Print and shaded views of the part. All mm, measured from the part's lowest x, y and z. A direction names the side the tool comes from. Give positions to 0.01 mm unless a question says otherwise; leave off trailing zeros. Write each loop counter-clockwise with the first axis right and the second up, starting at its lowest first coordinate (ties: lowest second). Pieces come first, ordered by that corner, then holes. Notation, with made-up numbers: (-18, 83) -> (27, 83) arc R25 ccw to (27, 119) -> close; hole circle Ø10 at (25, 30). An arc over 180 degrees is marked (long way). Put each result on its own line as item: value.
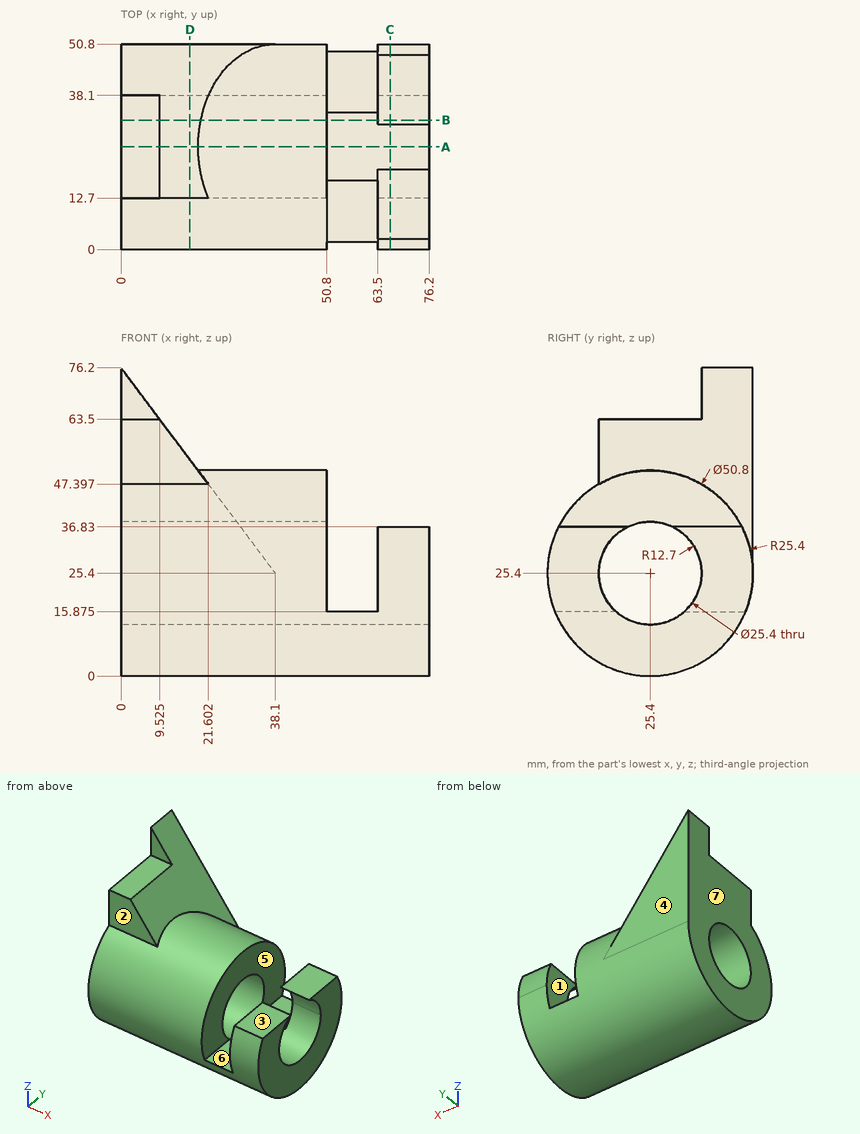
1) Slice it at A-A (y = 25.4). Write the cut outline in (x, z) (3 decimals), plus the area to 3 significant figures.
Filled sheet:
outline: (0, 0) -> (76.2, 0) -> (76.2, 12.7) -> (0, 12.7) -> close; (0, 38.1) -> (50.8, 38.1) -> (50.8, 50.8) -> (19.05, 50.8) -> (9.525, 63.5) -> (0, 63.5) -> close
area: 1,790 mm2
2) Slice it at D-D (x = 17). Write the cut outline in (y, z).
Filled sheet:
outline: (12.7, 47.4) arc R25.4 ccw (long way) to (50.8, 25.4) -> (50.8, 53.53) -> (12.7, 53.53) -> close; hole circle Ø25.4 at (25.4, 25.4)
3) Wall check: L1, parallel to X at y = 15, z = 35.5; L2, parallel to Z at x = 32, y = 25.4; L3, parallel to Y at x = 27, z = 25. Give the ranges that are in metal, low to high.
Filled sheet:
L1: 0 to 50.8, 63.5 to 76.2
L2: 0 to 12.7, 38.1 to 50.8
L3: 0 to 12.71, 38.09 to 50.8
4) Slice it at C-C (x = 66.5). Write the cut outline in (y, z).
Filled sheet:
outline: (2.72, 36.83) arc R25.4 ccw (long way) to (48.08, 36.83) -> (30.94, 36.83) arc R12.7 cw (long way) to (19.86, 36.83) -> close
5) Slice it at B-B (y = 32). Give the number of separate pieces and of enclosed holes in the cut face, plus the area to 3 significant figures.
Filled sheet:
separate pieces: 3
enclosed holes: 0
area: 1,940 mm2
6) Pin check, flat tips, straight feed: pin 1 (6.5 mm diameter, centred on x = 67.5, y = 8, fed in from +Z); pin 2 (1 mm diameter, centred on x = 29, y = 35.5, fed in from +Z); pin 3 (3 mm diameter, centred on x = 5.5, z = 71, fed in from -Y). Stop position of each tip, or through.
Filled sheet:
pin 1: z = 36.83
pin 2: z = 48.92
pin 3: y = 38.1
7) Pull direction X, two halves, no side cores. Call the marked faces 4, 5, 6 and 7: released by +X, released by -X, zero draft, split by the parting line, or undercut.
Filled sheet:
face 4: zero draft
face 5: undercut
face 6: undercut
face 7: released by -X
8) Tool access for the marked faces 1, 2 and 3: list every direction of +Z, -Z, +X, -X, +Y, -Y with a clear straight run to the whole face (end or side of a thin tool).
Filled sheet:
face 1: +Z, +Y, -Y
face 2: +Z, +X, -X, -Y
face 3: +Z, +X, +Y, -Y
